Check sheet for the modelled part. Datum: model origin and axes. Units: mm. Face numbers are marked on the shaded views. A direction names the side the tool comes from. Give positions to 0.01 mm unless a question says otherwise; leave off trailing zeros. Order: outer loops, then holes, each group sorted by start corner. A loop starts at its lowest first (then second) coordinate and runs counter-clockwise, first axis right, second up. Notation, with made-up numbers: (-15.5, 41) - (3.5, 41) arc R21 cw to (3.5, 73) - close; hole circle Ø3 at (16.5, -1.5). An arc over 180 degrees is marked (long way). Answer in a Markdown table with one row per item.
from build123d import *

# Parameters (mm, degrees)
BASE_EXTRUDE_DEPTH = 16


with BuildPart() as part:
    # Sketch1 → Base-Extrude (new body)
    with BuildSketch(Plane.XY):
        with BuildLine():
            Line((5.814342437, -160.974774553), (31.579798567, -151.59691545))
            ThreePointArc((31.579798567, -151.59691545), (40.735764364, -152.802321215), (45, -160.993841658))
            Line((45, -160.993841658), (45, -170.660453173))
            ThreePointArc((45, -170.660453173), (43.555274843, -175.838027157), (39.638545529, -179.519566863))
            Line((39.638545529, -179.519566863), (16.192727646, -191.79556845))
            ThreePointArc((16.192727646, -191.79556845), (-32.887869917, -190.276374217), (-57, -147.5))
            Line((-57, -147.5), (-57, -94.079804919))
            ThreePointArc((-57, -94.079804919), (-57.855513863, -81.027185697), (-60.407417371, -68.197900409))
            Line((-60.407417371, -68.197900409), (-73.410362798, -19.670247428))
            ThreePointArc((-73.410362798, -19.670247428), (-74.198496541, 16.449410659), (-58.219377677, 48.851858336))
            ThreePointArc((-58.219377677, 48.851858336), (-49.164213844, 54.989280966), (-38.234596516, 55.444707856))
            Line((-38.234596516, 55.444707856), (10.493757672, 43.759353856))
            ThreePointArc((10.493757672, 43.759353856), (44.773001659, 4.514235528), (19.017821778, -40.783850417))
            Line((19.017821778, -40.783850417), (0.321452148, -49.502110755))
            ThreePointArc((0.321452148, -49.502110755), (-12.301743374, -60.572356116), (-17, -76.691344366))
            Line((-17, -76.691344366), (-17, -145))
            ThreePointArc((-17, -145), (-9.750799418, -158.925584753), (5.814342437, -160.974774553))
        make_face()
        with BuildLine():
            Line((-15.821514229, -19.53382483), (-14.266024685, -17.978335287))
            ThreePointArc((-14.266024685, -17.978335287), (-14.009543632, -17.862047616), (-13.739996199, -17.943592295))
            ThreePointArc((-13.739996199, -17.943592295), (15.980613255, 15.980613255), (-17.943592295, -13.739996199))
            ThreePointArc((-17.943592295, -13.739996199), (-17.862047616, -14.009543632), (-17.978335287, -14.266024685))
            Line((-17.978335287, -14.266024685), (-19.53382483, -15.821514229))
            ThreePointArc((-19.53382483, -15.821514229), (-19.53382483, -19.53382483), (-15.821514229, -19.53382483))
        make_face(mode=Mode.SUBTRACT)
        with BuildLine():
            Line((-53, -8), (-56, -8))
            ThreePointArc((-56, -8), (-61.656854249, -5.656854249), (-64, 0))
            ThreePointArc((-64, 0), (-60.14032773, 21.889289173), (-49.02684436, 41.13840702))
            ThreePointArc((-49.02684436, 41.13840702), (-43.595734757, 43.965663727), (-37.756187937, 42.124461687))
            Line((-37.756187937, 42.124461687), (-35.458054608, 40.196098858))
            ThreePointArc((-35.458054608, 40.196098858), (-32.630797901, 34.764989255), (-34.47199994, 28.925442436))
            ThreePointArc((-34.47199994, 28.925442436), (-42.286167935, 15.39090645), (-45, 0))
            ThreePointArc((-45, 0), (-47.343145751, -5.656854249), (-53, -8))
        make_face(mode=Mode.SUBTRACT)
    extrude(amount=BASE_EXTRUDE_DEPTH)


solid = part.part
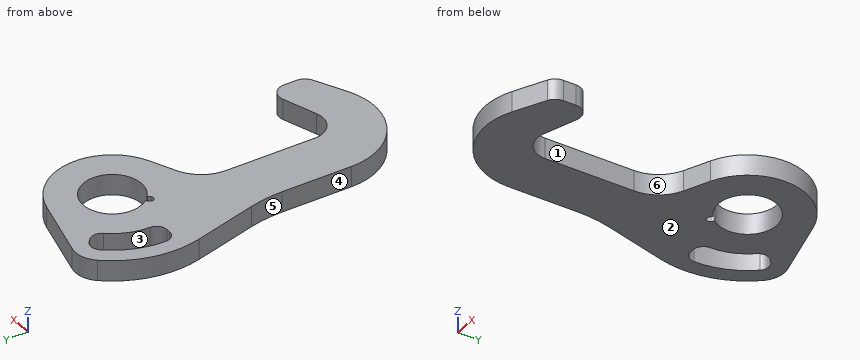
(1) Mould release check, pull along Y, two halves, no side actions. Record for the marked faces 4, 5 and 6: pulls with the +Y half, pulls with the -Y half, needs draft (parallel to the pull), parting line crosses it, or undercut.
Geometry says:
| item | result |
|---|---|
| face 4 | needs draft |
| face 5 | pulls with the -Y half |
| face 6 | undercut |
(2) Cross-section at B-B, the plane z = 5.25. Give the number of separate pieces and of enclosed holes in the cut face, then the cut area to 3 significant figures.
Geometry says:
| item | result |
|---|---|
| separate pieces | 1 |
| enclosed holes | 2 |
| area | 15,600 mm² |
(3) Access from +Z, -Z, +X, -X, +Y, -Y to the whole of each face (thin tool, end or side, straight path). Record for the marked faces 1, 2 and 3.
Geometry says:
| item | result |
|---|---|
| face 1 | +Z, -Z, +X |
| face 2 | -Z, +X, -X, +Y, -Y |
| face 3 | +Z, -Z |
(4) Cross-section at A-A, the plane x = 34.5. Record the cut outline in (y, z).
Geometry says:
| item | result |
|---|---|
| outline | (-182.21, 0) - (-151.01, 0) - (-151.01, 16) - (-182.21, 16) - close; (-28.89, 0) - (28.89, 0) - (28.89, 16) - (-28.89, 16) - close |
(5) Gauge pin test, flat ends, axial feed: P1, Ø6, axis at x = 2.5, z = 12.5, coming from the -Y side; P2, Ø5, axis at x = -58.5, y = -84.5, coming from the +Z side; P3, Ø1.5, axis at x = -32.5, z = 7.5, coming from the +Y side; P4, Ø5, axis at y = -58.5, z = 13, coming from the +X side. Record the tip position at first contact, or that the pin passes through.
Geometry says:
| item | result |
|---|---|
| P1 | y = -197.08 |
| P2 | z = 16 |
| P3 | y = 54.25 |
| P4 | x = -8.72 |
(6) Cross-section at D-D, the plane y = -97. Record the cut outline in (x, z), then the cut area to 3 significant figures.
Geometry says:
| item | result |
|---|---|
| outline | (-57, 0) - (-17, 0) - (-17, 16) - (-57, 16) - close |
| area | 640 mm² |
(7) Cross-section at C-C, the plane y = 2.5. Record the cut outline in (x, z), then the cut area to 3 significant figures.
Geometry says:
| item | result |
|---|---|
| outline | (-75.96, 0) - (-63.95, 0) - (-63.95, 16) - (-75.96, 16) - close; (-44.93, 0) - (-22.46, 0) - (-22.46, 16) - (-44.93, 16) - close; (22.46, 0) - (44.93, 0) - (44.93, 16) - (22.46, 16) - close |
| area | 911 mm² |
(8) Thickness scan on L1, parallel to Y at x = 0, z = 7.5; L2, parallel to Y at x = -9.5, z = 2.75; L3, parallel to X at y = -20, z = 8.75. Record the ranges inside material, lowest first.
Geometry says:
| item | result |
|---|---|
| L1 | -197.01 to -162, -49.65 to -22.6, 22.6 to 46.28 |
| L2 | -197.44 to -159.1, -56.85 to -20.51, 20.51 to 48.55 |
| L3 | -73.32 to -18.9, -16.45 to -10.52, 10.52 to 40.31 |
